Autodesk Inventor part; units mm, degrees
ref_plane "YZ Plane" through (0, 0, 0) normal (1, 0, 0) x (0, 1, 0)
ref_plane "XZ Plane" through (0, 0, 0) normal (0, 1, 0) x (-1, 0, 0)
ref_plane "XY Plane" through (0, 0, 0) normal (0, 0, 1) x (1, 0, 0)
sketch "Sketch1" plane through (0, 0, 0) normal (1, 0, 0) x (0, 1, 0)
  line L0 (2, 0) -> (18, 0)
  line L1 (20, -2) -> (20, -18)
  line L2 (18, -20) -> (2, -20)
  line L3 (0, -18) -> (0, -2)
  line L4 (18, -18) -> (18, -2)
  line L5 (18, -2) -> (2, -2)
  line L6 (2, -2) -> (2, -18)
  line L7 (2, -18) -> (18, -18)
  arc A0 (20, -2) -> (18, 0) centre (18, -2) ccw
  arc A1 (18, -20) -> (20, -18) centre (18, -18) ccw
  arc A2 (0, -18) -> (2, -20) centre (2, -18) ccw
  arc A3 (2, 0) -> (0, -2) centre (2, -2) ccw
  point P0 (0, 0)
  point P1 (20, -20)
  point P2 (20, 0)
  point P3 (0, -20)
  dimension "d0" = 20
  dimension "d1" = 20
  dimension "d2" = 2
  dimension "d5" = 2
extrude "Extrusion1" add sketch "Sketch1" along normal blind 319
sketch "Sketch2" plane through (0, 0, -18) normal (0, -1, 0) x (1, 0, 0)
  line L0 (0, 16) -> (0, 0)
  line L1 (0, 0) -> (319, 0)
  point P0 (0, 18)
  point P1 (16, 8)
  dimension "d6" = 16
  dimension "d7" = 8
hole "Hole1" at (16, 0, -10) direction (0, 1, 0) diameter 2.45 depth 2
sketch "Sketch4" plane through (0, 2, -20) normal (0, 0, -1) x (-1, 0, 0)
  line L0 (0, 0) -> (0, 16)
  line L1 (0, 16) -> (-319, 16)
  line L2 (0, 0) -> (-16, 0)
  line L3 (-16, 0) -> (-16, 16)
  line L4 (-16, 16) -> (0, 16)
  line L5 (0, 16) -> (0, 0)
  circle A0 centre (-8, 8) radius 8
  circle A1 centre (-8, 8) radius 5
  circle A2 centre (-8, 8) radius 6.5
  line L6 (0, 18) -> (-319, 18)
  line L7 (-2.6429, 18) -> (0, 16.4741)
  line L8 (-2.6429, 18) -> (-0.6491, 18) construction
  line L9 (0, 18) -> (0, 16)
  point P0 (0, -2)
  point P1 (-8, 1.5)
  point P2 (-1.5, 8)
  point P3 (-8, 14.5)
  point P4 (-14.5, 8)
  dimension "d21" = 10
  dimension "d22" = 13
  dimension "d30" = 30
  dimension "d33" = 2.6429
extrude "Extrusion3" cut sketch "Sketch4" against normal up to surface (2 mm away) contours A1
hole "Hole2" at (8, 3.5, -20) at (1.5, 10, -20) at (14.5, 10, -20) at (8, 16.5, -20) direction (0, 0, 1) diameter 2 end through all
extrude "Extrusion4" cut sketch "Sketch4" against normal up to next contours L7 L6 L9
properties part number "rockerpivotarm"
For this review, take the finished solid that the model builds, in its own axes (mm). A direction names the side the tool comes from. Coordinates: 2 decimals unless noted, no trailing zeros. Loops run counter-clockwise (first coordinate to the right, second up) from the corner with the lowest first, then second, coordinate; pieces in that order, holes last. Notation, with made-up numbers: (55, 0) -> (98, 0) arc R27 ccw to (98, 38) -> close; hole circle Ø8 at (85.25, 4.25). An arc over 180 degrees is marked (long way). Return JSON: item names as keys, results as strings. Group by question number.
(1) Consider section A-A, the plane x = 153. Give the boundary of the cut face in (y, z), plus the area to 3 significant figures.
(2) Mouldability with a two-part tool opening along Z and no side actions: class faces 1 (the flat face through (157, 10, 0)), 2 (the flat face through (157, 10, -2)), 3 (the flat face through (0, 1.7, -10)) as pulls with the +Z half, pulls with the -Z half, needs draft (parallel to the pull), parting line crosses it, or undercut.
(3) To check wall thickness, follow L1, parallel to X at y = 10, z = -0.85; L2, parallel to Y at x = 8, z = -1.5; L3, parallel to Z at x = 95, y = 16. State the ranges of each line that lie inside material, in increasing order.
(4) For pin 1 Ø2 at (x, z) = (16, -10) entering from -Y; pin 2 Ø9 at (x, y) = (8, 10) entering from -Z, all flat-tipped, find the tip position at first contact; note any pin that passes through.
(5) Tool access review of faces 4 (the flat face through (157, 10, -18)), 5 (the flat face through (157, 0, -10)), 6 (the cylindrical face through (3.23, 11.5, -19.01)): name each direction out of +Z, -Z, +X, -X, +Y, -Y from which nothing blocks a thin tool from reaching the whole face with its end or side.
Results below:
{
 "1": {"outline": "(0, -18) arc R2 ccw to (2, -20) -> (18, -20) arc R2 ccw to (20, -18) -> (20, -2) arc R2 ccw to (18, 0) -> (2, 0) arc R2 ccw to (0, -2) -> close; hole (2, -18) -> (18, -18) -> (18, -2) -> (2, -2) -> close", "area": "141 mm2"},
 "2": {"face 1": "pulls with the +Z half", "face 2": "undercut", "face 3": "needs draft"},
 "3": {"L1": "x = 0 to 0.5, 2.5 to 13.5, 15.5 to 319", "L2": "y = 0.06 to 2.5, 4.5 to 15.5, 17.5 to 19.94", "L3": "z = -20 to -18, -2 to 0"},
 "4": {"pin 1": "stops at y = 18", "pin 2": "stops at z = -2"},
 "5": {"face 4": "+X, -X", "face 5": "+Z, -Z, +X, -X, -Y", "face 6": "-Z"}
}
